Design review of the part shown in the three views and the two pictorial views. Dimensions are in mm from the part's minimum x, y and z. A direction names the side the tool comes from. Give positions to 0.01 mm unless a question says otherwise; leave off trailing zeros. Write each loop counter-clockwise with the first axis right and the second up, starting at its lowest first coordinate (ties: lowest second). Pieces come first, ordered by that corner, then holes. Notation, with made-up numbers: M 74,73 L 123,73 A21 ccw 123,95 Z; hole C 39.5,-33 d4. An arc over 180 degrees is marked long. Write item = value, one per line.
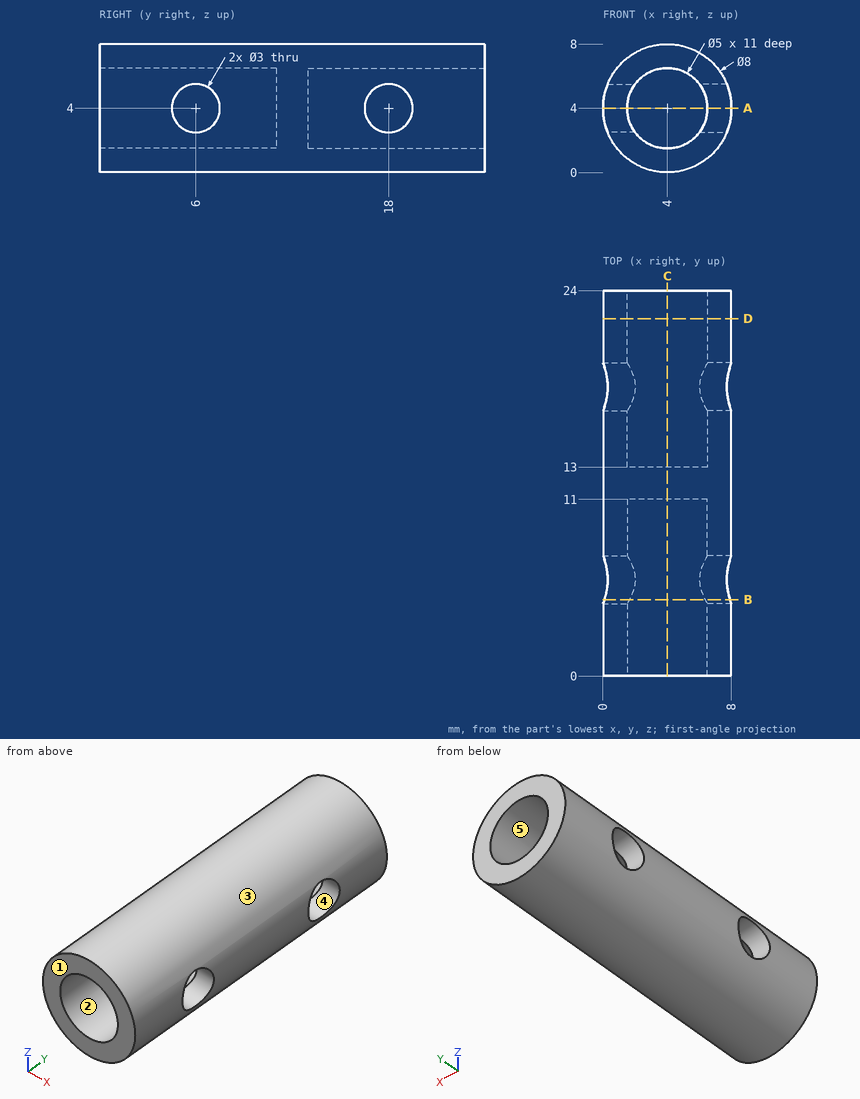
1. We need section B-B, the plane y = 4.75. Write out the cut boundary in (x, z).
Responses:
outline = M 0.09,3.17 A4 ccw 7.91,3.17 L 6.36,3.17 A2.5 cw 1.64,3.17 Z; M 0.09,4.83 L 1.64,4.83 A2.5 cw 6.36,4.83 L 7.91,4.83 A4 ccw Z
2. For line 1 along Y through (x, z) = (0.75, 5.25); line 2 along X through (y, z) = (19, 2.5); line 3 along X through (y, z) = (4.25, 6), list the stretches that pass through material, from the lowest coordinate up. Write a range as from..to.
Responses:
line_1 = 0..5.17, 6.83..17.17, 18.83..24
line_2 = 0.29..2, 6..7.71
line_3 = 0.54..2.5, 5.5..7.46
3. Insertion check: P1, Ø2.5, axis at y = 18, z = 4, coming from the -X side. The pin has a flat end and moves straight along its axis. Give the tip position at first contact, or say it passes through.
Responses:
P1 = through
4. The part is to be moulded in two halves that separate along X. For the marked faces 1, 2 and 3, say which applies: +X half, -X half, draft (parallel to the pull), parting line (faces both ways), or undercut.
Responses:
face_1 = draft
face_2 = undercut
face_3 = parting line
5. We need section C-C, the plane x = 4. Write out the cut boundary in (y, z), then the cut area to 3 significant figures.
Responses:
outline = M 0,0 L 24,0 L 24,1.5 L 13,1.5 L 13,6.5 L 24,6.5 L 24,8 L 0,8 L 0,6.5 L 11,6.5 L 11,1.5 L 0,1.5 Z
area = 82.0 mm2
6. Machinability: for the marked faces 4 and 5, which of the approach directions +Z, -Z, +X, -X, +Y, -Y give a long, thin tool a straight path to every point of the face, cutting with its end or side? Answer none if there is none.
Responses:
face_4 = +X, -X
face_5 = +Y
7. We need section D-D, the plane y = 22.25. Write out the cut boundary in (x, z).
Responses:
outline = C 4,4 d8; hole C 4,4 d5
8. We need section A-A, the plane z = 4. Write out the cut boundary in (x, y), then the cut area to 3 significant figures.
Responses:
outline = M 0,0 L 1.5,0 L 1.5,4.5 L 0,4.5 Z; M 0,7.5 L 1.5,7.5 L 1.5,11 L 6.5,11 L 6.5,7.5 L 8,7.5 L 8,16.5 L 6.5,16.5 L 6.5,13 L 1.5,13 L 1.5,16.5 L 0,16.5 Z; M 0,19.5 L 1.5,19.5 L 1.5,24 L 0,24 Z; M 6.5,0 L 8,0 L 8,4.5 L 6.5,4.5 Z; M 6.5,19.5 L 8,19.5 L 8,24 L 6.5,24 Z
area = 64.0 mm2
